```python
from build123d import *

# Parameters (mm, degrees)
F0_W     = 87.4
F0_H     = 57.4
F1_DEPTH = 10
F2_R     = 5
F3_T     = -1.2


with BuildPart() as f1:
    # F0 (on Top) → F1 (new body)
    with BuildSketch(Plane.XY):
        Rectangle(F0_W, F0_H)
    extrude(amount=F1_DEPTH)

    # F2
    f2_edges = [f1.edges().sort_by_distance(p)[0] for p in [
        (43.7, -28.7, 5),
        (43.7, 28.7, 5),
        (-43.7, 28.7, 5),
        (-43.7, -28.7, 5),
        (-43.7, 0, 0),
        (0, 28.7, 0),
        (0, -28.7, 0),
        (43.7, 0, 0),
    ]]
    fillet(f2_edges, radius=F2_R)

    # F3
    f3_openings = [f1.faces().sort_by_distance(p)[0] for p in [
        (0, 0, 10),
    ]]
    offset(amount=F3_T, openings=f3_openings)


solid = f1.part
```
Could you check a few things on this model? Use its own coordinates, in mm. A direction names the side the tool comes from. Coordinates: 2 decimals unless noted, no trailing zeros. Loops run counter-clockwise (first coordinate to the right, second up) from the corner with the lowest first, then second, coordinate; pieces in that order, holes last. Notation, with made-up numbers: M 4.25,-7.5 L 49.25,-7.5 A15 cw 49.25,0.5 Z; hole C -6,55.5 d8. An arc over 180 degrees is marked long. Put each result on its own line as item: value. Start each with the question number.
(1) Suppose I cut it at C-C on x = 31. Please give me the cut outline in (y, z).
(2) Thinking about a two-plate mould opening in Y: for faces 1 (the face through (0.542, 26.416, 2.343)), 2 (the face through (-42.27, 0.33, 1.5)), 3 (the face through (-1, 28.7, 7)), which applies, pulls with the +Y half, pulls with the -Y half, needs draft (parallel to the pull), parting line crosses it, or undercut?
(3) I need wall thicknesses on line 1 (Y direction, x = 2.5, z = 5.5); line 2 (X direction, y = 23.5, z = 8); line 3 (Z direction, x = -4, y = -24). Which ranges of each line are inside material? Lowest first, please. Write a range as from..to.
(4) Will these pins go through, and if not, where does the flat tip stop? P1, Ø1, axis at x = 6, y = -19.5, coming from the +Z side; P2, Ø3, axis at x = -33.5, z = 2.5, coming from the -Y side.
(5) Suppose I cut it at A-A on y = -22. Please give me the cut outline in (x, z), then the cut area to 3 significant figures.
(6) For faces 4 (the face through (-42.5, 0, 7)), 5 (the face through (0.54, 27.27, 1.5)), which set-ups out of +Z, -Z, +X, -X, +Y, -Y let a thin tool reach every point of the face, with its end or its side?
(7) Suppose I cut it at D-D on z = 2.5. Please give me the cut outline in (x, y).
(8) Suppose I cut it at B-B on z = 8.5. Please give me the cut outline in (x, y), then the cut area to 3 significant figures.
Solutions:
1. outline: M -28.7,5 A5 ccw -23.7,0 L 23.7,0 A5 ccw 28.7,5 L 28.7,10 L 27.5,10 L 27.5,5 A3.8 cw 23.7,1.2 L -23.7,1.2 A3.8 cw -27.5,5 L -27.5,10 L -28.7,10 Z
2. face 1: undercut
2. face 2: needs draft
2. face 3: pulls with the +Y half
3. line 1: y = -28.7..-27.5, 27.5..28.7
3. line 2: x = -43.7..-42.5, 42.5..43.7
3. line 3: z = 0.01..1.21
4. P1: stops at z = 1.2
4. P2: stops at y = -28.6
5. outline: M -43.7,5 A5 ccw -38.7,0 L 38.7,0 A5 ccw 43.7,5 L 43.7,10 L 42.5,10 L 42.5,5 A3.8 cw 38.7,1.2 L -38.7,1.2 A3.8 cw -42.5,5 L -42.5,10 L -43.7,10 Z
5. area: 121 mm2
6. face 4: +Z
6. face 5: -Z, +X, -X, +Y
7. outline: M -43.03,-23.7 A4.33 ccw -38.7,-28.03 L 38.7,-28.03 A4.33 ccw 43.03,-23.7 L 43.03,23.7 A4.33 ccw 38.7,28.03 L -38.7,28.03 A4.33 ccw -43.03,23.7 Z; hole M -41.56,-23.7 A2.86 ccw -38.7,-26.56 L 38.7,-26.56 A2.86 ccw 41.56,-23.7 L 41.56,23.7 A2.86 ccw 38.7,26.56 L -38.7,26.56 A2.86 ccw -41.56,23.7 Z
8. outline: M -43.7,-23.7 A5 ccw -38.7,-28.7 L 38.7,-28.7 A5 ccw 43.7,-23.7 L 43.7,23.7 A5 ccw 38.7,28.7 L -38.7,28.7 A5 ccw -43.7,23.7 Z; hole M -42.5,-23.7 A3.8 ccw -38.7,-27.5 L 38.7,-27.5 A3.8 ccw 42.5,-23.7 L 42.5,23.7 A3.8 ccw 38.7,27.5 L -38.7,27.5 A3.8 ccw -42.5,23.7 Z
8. area: 333 mm2
